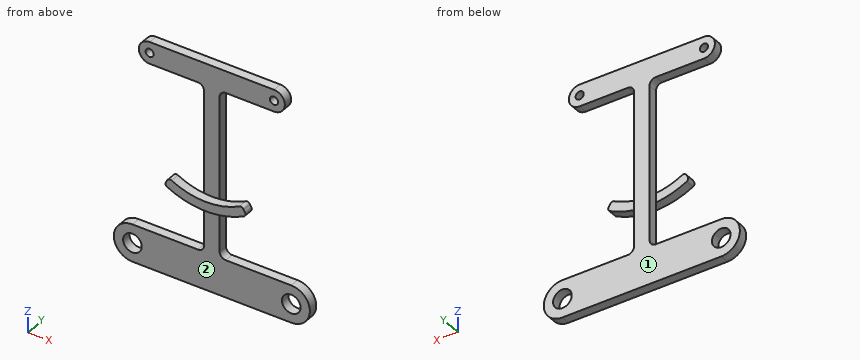
```python
from build123d import *

# Parameters (mm, degrees)
SKETCH1_R           = 1.3
SKETCH1_R_2         = 3
BOSS_EXTRUDE4_DEPTH = 3
BOSS_EXTRUDE5_DEPTH = 3
FILLET4_R           = 1
FILLET5_R           = 2


with BuildPart() as part:
    # Sketch1 → Boss-Extrude4 (new body)
    with BuildSketch(Plane(origin=(0, 0, 0), x_dir=(1, 0, 0), z_dir=(0, 1, 0))):
        with BuildLine():
            Line((-25.55, 54.240000374), (25.55, 54.240000374))
            ThreePointArc((25.55, 54.240000374), (31.550000374, 48.24), (25.55, 42.239999626))
            Line((25.55, 42.239999626), (2.5, 42.239999626))
            Line((2.5, 42.239999626), (2.5, -11.500002156))
            Line((2.5, -11.500002156), (20, -11.500003832))
            ThreePointArc((20, -11.500003832), (23.499996168, -15), (20, -18.499996168))
            Line((20, -18.499996168), (-20, -18.5))
            ThreePointArc((-20, -18.5), (-23.5, -15), (-20, -11.5))
            Line((-20, -11.5), (-2.5, -11.500001677))
            Line((-2.5, -11.500001677), (-2.5, 42.239999626))
            Line((-2.5, 42.239999626), (-25.55, 42.239999626))
            ThreePointArc((-25.55, 42.239999626), (-31.550000374, 48.24), (-25.55, 54.240000374))
        make_face()
        with Locations(Location((-20, -15, 0), (0, 0, 270))):
            Circle(SKETCH1_R, mode=Mode.SUBTRACT)
        with Locations(Location((20, -15, 0), (0, 0, 270))):
            Circle(SKETCH1_R, mode=Mode.SUBTRACT)
        with Locations(Location((25.55, 48.24, 0), (0, 0, 270))):
            Circle(SKETCH1_R_2, mode=Mode.SUBTRACT)
        with Locations(Location((-25.55, 48.24, 0), (0, 0, 270))):
            Circle(SKETCH1_R_2, mode=Mode.SUBTRACT)
    extrude(amount=BOSS_EXTRUDE4_DEPTH)

    # Sketch2 → Boss-Extrude5 (add)
    with BuildSketch(Plane(origin=(0, 0, 0), x_dir=(1, 0, 0), z_dir=(0, 1, 0))):
        with BuildLine():
            Line((-11.75, 20.351596989), (-13.25, 22.9496732))
            ThreePointArc((-13.25, 22.9496732), (0, 26.5), (13.25, 22.9496732))
            Line((13.25, 22.9496732), (11.75, 20.351596989))
            ThreePointArc((11.75, 20.351596989), (0, 23.5), (-11.75, 20.351596989))
        make_face()
    extrude(amount=-BOSS_EXTRUDE5_DEPTH)

    # Fillet4
    fillet4_edges = [part.edges().sort_by_distance(p)[0] for p in [
        (-13.25, -1.5, -22.9496732),
        (13.25, -1.5, -22.9496732),
        (11.75, -1.5, -20.351596989),
        (-11.75, -1.5, -20.351596989),
    ]]
    fillet(fillet4_edges, radius=FILLET4_R)

    # Fillet5
    fillet5_edges = [part.edges().sort_by_distance(p)[0] for p in [
        (-2.5, 1.5, 11.500001677),
        (-2.5, 1.5, -42.239999626),
        (2.5, 1.5, -42.239999626),
        (2.5, 1.5, 11.500002156),
    ]]
    fillet(fillet5_edges, radius=FILLET5_R)


solid = part.part
```
Source: CAD feature listing. Evaluate the final solid. Frame: model axes, mm. Face numbers are marked on the shaded views. A direction names the side the tool comes from. Round coordinates to 2 decimals unless told otherwise and drop trailing zeros. Loops run counter-clockwise (first coordinate to the right, second up) from the corner with the lowest first, then second, coordinate; pieces in that order, holes last. Notation, with made-up numbers: M 78.5,2 L 133.5,2 A32 ccw 133.5,32 Z; hole C 5.25,58 d2. An arc over 180 degrees is marked long. Use a Markdown table: item, result. Add a question column.
1. Cut plane D-D, the plane z = 6. Output: boundary loops of the cut face in (x, y), and give its area (3 significant figures).
2. Set-up query: the marked faces 1 and 2. Return all of +Z, -Z, +X, -X, +Y, -Y with unobstructed straight access to the full face (end or side cutting, diameter ignored); none if empty.
3. Contact query for flat-ended pins moving along their axis: pin 1 (8 mm diameter, centred on x = 14.5, z = -39.5, fed in from +Y); pin 2 (21 mm diameter, centred on x = -10, z = 0.5, fed in from -Y); pin 3 (3.5 mm diameter, centred on x = -25.55, z = -48.24, fed in from -Y); pin 4 (1.5 mm diameter, centred on y = 1.5, z = -24.5, fed in from -X). Output: stop coordinate, or through.
4. Cut plane C-C, the plane x = -0.5. Output: boundary loops of the cut face in (y, z).
5. Ray query, line 1 along X through (y, z) = (2.1, -48.24); line 2 along X through (y, z) = (1.7, 15); line 3 along Z through (x, y) = (-6.5, 2.45). Return the intervals inside material, ascending. Write a range as [from, to].
6. Cut plane B-B, the plane y = 1.5. Output: boundary loops of the cut face in (x, z).
7. Cut plane A-A, the plane z = -48.24. Output: boundary loops of the cut face in (x, y).
Solution:
| question | item | result |
|---|---|---|
| 1 | outline | M -2.5,0 L 2.5,0 L 2.5,3 L -2.5,3 Z |
| 1 | area | 15.0 mm2 |
| 2 | face 1 | +Z, -Z, +X, -X, +Y |
| 2 | face 2 | -Z, +X, -X, -Y |
| 3 | pin 1 | stops at y = 3 |
| 3 | pin 2 | stops at y = 0 |
| 3 | pin 3 | passes through |
| 3 | pin 4 | stops at x = -2.5 |
| 4 | outline | M -3,-26.5 L 0,-26.5 L 0,-54.24 L 3,-54.24 L 3,18.5 L 0,18.5 L 0,-23.49 L -3,-23.49 Z |
| 5 | line 1 | x = [-31.55, -28.55], [-22.55, 22.55], [28.55, 31.55] |
| 5 | line 2 | x = [-23.5, -21.3], [-18.7, 18.7], [21.3, 23.5] |
| 5 | line 3 | z = [-54.24, -42.24], [11.5, 18.5] |
| 6 | outline | M -25.55,-54.24 L 25.55,-54.24 A6 ccw 25.55,-42.24 L 4.5,-42.24 A2 cw 2.5,-40.24 L 2.5,9.5 A2 cw 4.5,11.5 L 20,11.5 A3.5 ccw 20,18.5 L -20,18.5 A3.5 ccw -20,11.5 L -4.5,11.5 A2 cw -2.5,9.5 L -2.5,-40.24 A2 cw -4.5,-42.24 L -25.55,-42.24 A6 ccw Z; hole C -25.55,-48.24 d6; hole C -20,15 d2.6; hole C 20,15 d2.6; hole C 25.55,-48.24 d6 |
| 7 | outline | M -31.55,0 L -28.55,0 L -28.55,3 L -31.55,3 Z; M -22.55,0 L 22.55,0 L 22.55,3 L -22.55,3 Z; M 28.55,0 L 31.55,0 L 31.55,3 L 28.55,3 Z |
